Answer from the drawing. Dimensions are ordinates in mm from the lowest x, y and z of the part. A direction names the side the tool comes from. Coordinates: 2 decimals unless noted, no trailing zeros. Write each loop counter-clockwise with the first axis right and the second up, starting at its lowest first coordinate (ties: lowest second). Pieces come first, ordered by that corner, then holes.
(1) For a pull along X with two mould halves and no side action, classify the marked faces 1, 2, 3 and 4 as +X half, -X half, draft (parallel to the pull), parting line (faces both ways), or undercut.
(2) The part is cut by section D-D on y = 1.35. Determine the outline of the cut face in (x, z), plus the area to 3 significant figures.
(3) Straight lines are drawn through the part: line 1 (X direction, y = 0.5, z = 16.25); line 2 (Y direction, x = 17.75, z = 10.75). For each, find the intervals that lie inside material, in ascending order.
(4) The part is cut by section C-C on y = 2.65. Determine the outline of the cut face in (x, z), plus the area to 3 significant figures.
(5) The part is cut by section B-B on z = 14.25. Determine the outline of the cut face in (x, y), plus the area to 3 significant figures.
(6) Which of the six approach directions +Z, -Z, +X, -X, +Y, -Y give full straight-line access (tool end or side, diameter ignored) to the marked faces 5 and 6?
(7) The part is cut by section A-A on x = 14.5. Determine the outline of the cut face in (y, z).
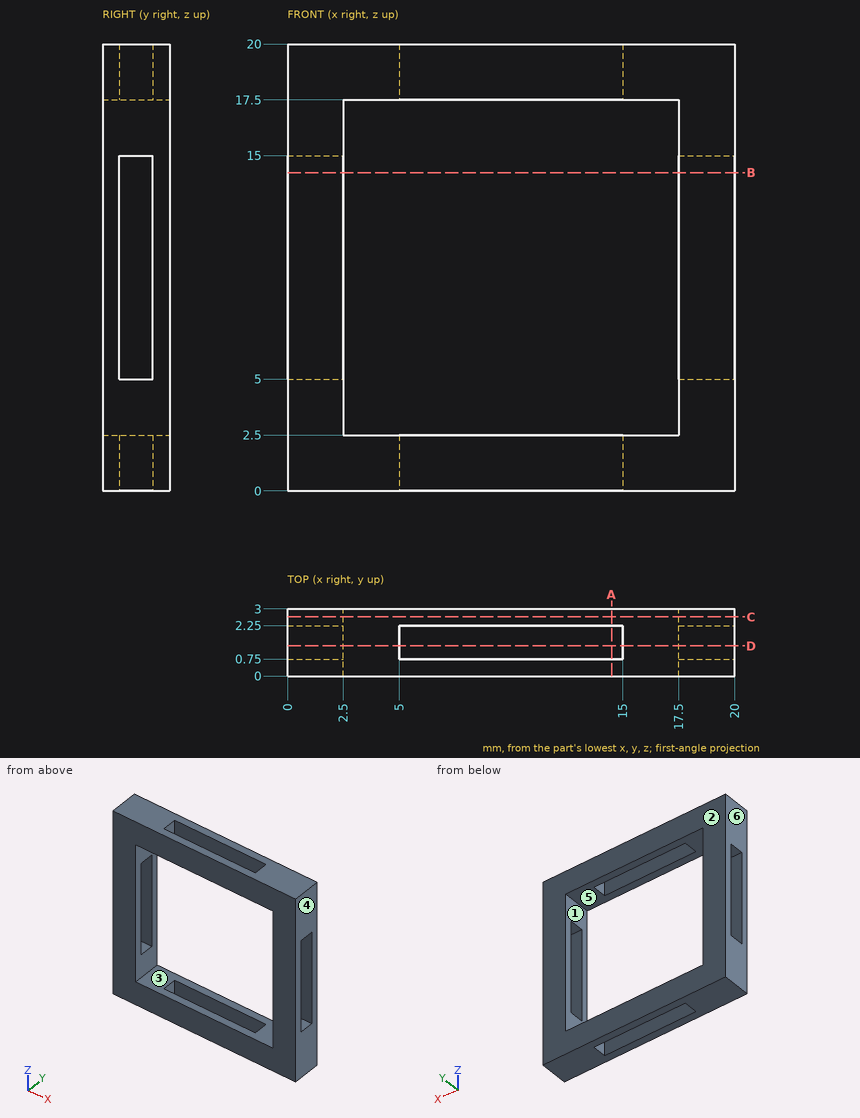
Model answer:
1. face 1: undercut
1. face 2: draft
1. face 3: undercut
1. face 4: +X half
2. outline: (0, 0) - (5, 0) - (5, 2.5) - (2.5, 2.5) - (2.5, 5) - (0, 5) - close; (0, 15) - (2.5, 15) - (2.5, 17.5) - (5, 17.5) - (5, 20) - (0, 20) - close; (15, 0) - (20, 0) - (20, 5) - (17.5, 5) - (17.5, 2.5) - (15, 2.5) - close; (15, 17.5) - (17.5, 17.5) - (17.5, 15) - (20, 15) - (20, 20) - (15, 20) - close
2. area: 75.0 mm2
3. line 1: x = 0 to 2.5, 17.5 to 20
3. line 2: y = 0 to 0.75, 2.25 to 3
4. outline: (0, 0) - (20, 0) - (20, 20) - (0, 20) - close; hole (2.5, 2.5) - (17.5, 2.5) - (17.5, 17.5) - (2.5, 17.5) - close
4. area: 175 mm2
5. outline: (0, 0) - (2.5, 0) - (2.5, 0.75) - (0, 0.75) - close; (0, 2.25) - (2.5, 2.25) - (2.5, 3) - (0, 3) - close; (17.5, 0) - (20, 0) - (20, 0.75) - (17.5, 0.75) - close; (17.5, 2.25) - (20, 2.25) - (20, 3) - (17.5, 3) - close
5. area: 7.50 mm2
6. face 5: +Y, -Y
6. face 6: +Z, -Z, -X, +Y, -Y
7. outline: (0, 0) - (0.75, 0) - (0.75, 2.5) - (0, 2.5) - close; (0, 17.5) - (0.75, 17.5) - (0.75, 20) - (0, 20) - close; (2.25, 0) - (3, 0) - (3, 2.5) - (2.25, 2.5) - close; (2.25, 17.5) - (3, 17.5) - (3, 20) - (2.25, 20) - close
